Design review of the part built by this model. Coordinates are the model's own, in mm. Face numbers are marked on the shaded views. Coordinates: 2 decimals unless noted, no trailing zeros. Loops run counter-clockwise (first coordinate to the right, second up) from the corner with the lowest first, then second, coordinate; pieces in that order, holes last. Notation, with made-up numbers: M 89,-31 L 97,-31 A20 ccw 97,7 Z; hole C -37.5,61.25 d4. An arc over 180 degrees is marked long. Write item = value, one per line. Start each with the question number.
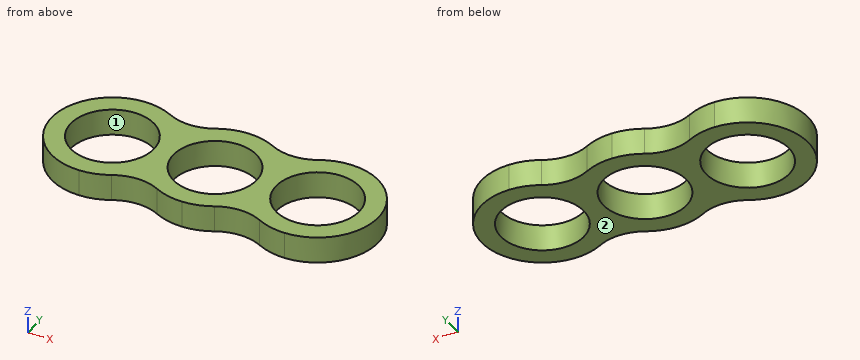
```python
from build123d import *

# Parameters (mm, degrees)
F0_R     = 11
F1_DEPTH = 7
F2_R     = 12.7


with BuildPart() as f1:
    # F0 (on Top) → F1 (new body)
    with BuildSketch(Plane.XY):
        with BuildLine():
            ThreePointArc((-27.08, 16.08), (-43.16, 0), (-27.08, -16.08))
            ThreePointArc((-27.08, -16.08), (-19.363404, -14.107464), (-13.54, -8.6738))
            ThreePointArc((-13.54, -8.6738), (-7.716596, -14.107464), (0, -16.08))
            ThreePointArc((0, -16.08), (7.716596, -14.107464), (13.54, -8.6738))
            ThreePointArc((13.54, -8.6738), (19.363404, -14.107464), (27.08, -16.08))
            ThreePointArc((27.08, -16.08), (43.16, 0), (27.08, 16.08))
            ThreePointArc((27.08, 16.08), (19.363404, 14.107464), (13.54, 8.6738))
            ThreePointArc((13.54, 8.6738), (7.716596, 14.107464), (0, 16.08))
            ThreePointArc((0, 16.08), (-7.716596, 14.107464), (-13.54, 8.6738))
            ThreePointArc((-13.54, 8.6738), (-19.363404, 14.107464), (-27.08, 16.08))
        make_face()
        with Locations((-27.08, 0)):
            Circle(F0_R, mode=Mode.SUBTRACT)
        with BuildLine():
            ThreePointArc((0, -11), (-11, 0), (0, 11))
            ThreePointArc((0, 11), (11, 0), (0, -11))
        make_face(mode=Mode.SUBTRACT)
        with Locations((27.08, 0)):
            Circle(F0_R, mode=Mode.SUBTRACT)
    extrude(amount=F1_DEPTH)

    # F2
    f2_edges = [f1.edges().sort_by_distance(p)[0] for p in [
        (-13.54, -8.6738, 3.5),
        (13.54, -8.6738, 3.5),
        (-13.54, 8.6738, 3.5),
        (13.54, 8.6738, 3.5),
    ]]
    fillet(f2_edges, radius=F2_R)


solid = f1.part
```
(1) Take a section at A-A (y = 0). State the section outline as (x, z) points, plus the area to 3 significant figures.
(2) Mouldability with a two-part tool opening along X and no side actions: class the marked faces 1 and 2 as +X half, -X half, draft (parallel to the pull), parting line (faces both ways), or undercut.
(3) Take a section at B-B (x = 31). State the section outline as (y, z) points, plus the area to 3 significant figures.
(4) Insertion check: pin 1 (1 mm diameter, centred on y = 8, z = 1.5, fed in from -X); pin 2 (1.5 mm diameter, centred on x = -11.5, z = 3.5, fed in from -Y); pin 3 (17.5 mm diameter, centred on x = 27.08, y = 0, fed in from -Z); pin 4 (1 mm diameter, centred on x = -25, z = 3.5, fed in from -Y). Each pin has a flat end and moves straight along its axis. Give the tip position at first contact, or say it passes through.
(5) To check wall thickness, follow L1, parallel to X at y = -6.5, z = 5.75; L2, parallel to X at y = -9, z = 5; L3, parallel to Y at x = 27.08, z = 5.5. State the ranges of each line that lie inside material, in increasing order.
(6) Take a section at D-D (y = -4.5). State the section outline as (x, z) points.
(7) Take a section at C-C (z = 4). Give the number of separate pieces and of enclosed holes in the cut face, plus the area to 3 significant figures.
Results list:
q1.outline = M -43.16,0 L -38.08,0 L -38.08,7 L -43.16,7 Z; M -16.08,0 L -11,0 L -11,7 L -16.08,7 Z; M 11,0 L 16.08,0 L 16.08,7 L 11,7 Z; M 38.08,0 L 43.16,0 L 43.16,7 L 38.08,7 Z
q1.area = 142 mm^2
q2.face_1 = undercut
q2.face_2 = draft
q3.outline = M -15.59,0 L -10.28,0 L -10.28,7 L -15.59,7 Z; M 10.28,0 L 15.59,0 L 15.59,7 L 10.28,7 Z
q3.area = 74.4 mm^2
q4.pin_1 = -41.3
q4.pin_2 = -13.01
q4.pin_3 = through
q4.pin_4 = -16
q5.L1 = -41.79 to -35.95, -18.21 to -8.87, 8.87 to 18.21, 35.95 to 41.79
q5.L2 = -40.41 to -33.4, -20.76 to -6.32, 6.32 to 20.76, 33.4 to 40.41
q5.L3 = -16.08 to -11, 11 to 16.08
q6.outline = M -42.52,0 L -37.12,0 L -37.12,7 L -42.52,7 Z; M -17.04,0 L -10.04,0 L -10.04,7 L -17.04,7 Z; M 10.04,0 L 17.04,0 L 17.04,7 L 10.04,7 Z; M 37.12,0 L 42.52,0 L 42.52,7 L 37.12,7 Z
q7.separate_pieces = 1
q7.enclosed_holes = 3
q7.area = 1,240 mm^2
